Part model, mm, in its own coordinate system. A direction names the side the tool comes from. Round coordinates to 2 decimals unless told otherwise and drop trailing zeros. Order: outer loops, then holes, each group sorted by start corner. A loop starts at its lowest first (then second) coordinate and runs counter-clockwise, first axis right, second up. Notation, with made-up numbers: (-36, 13.5) - (2, 13.5) arc R13 ccw to (2, 17.5) - close; hole circle Ø10 at (21, -1). An arc over 180 degrees is marked (long way). Return JSON: item names as keys, results as strings. Group by question number.
Item 1: Saw through at B-B on z = -0.85. State how many separate pieces and enclosed holes the cut face has, and give its area (3 significant figures).
Item 2: Tool access for faces 5 (the face through (33, 0, -1.25)), 6 (the face through (78.29, 10.97, -0.02)): list every direction of +Z, -Z, +X, -X, +Y, -Y with a clear straight run to the whole face (end or side of a thin tool).
Item 3: Saw through at A-A on x = 100. List the corners of the cut face in (y, z), and give its area (3 significant figures).
Item 4: Probe probe 1 along X at (y, z) = (-7, -0.4); probe 2 along X at (y, z) = (-4, 0.95); probe 3 along Y at (x, z) = (108.5, -0.45). List the from-to ranges inside material, lowest first.
Item 5: Two-plate mould, pull along X, no slides. Class faces 1 (the face through (78.29, -10.97, -0.02)), 2 (the face through (-111.108, -0.319, 0.018)), 3 (the face through (4, 0, 1.25)), 4 (the face through (122.487, 0.771, 0.018)): released by +X, released by -X, zero draft, split by the parting line, or undercut.
Item 6: Drop flat-ended pins along their axis: pin 1 (2.5 mm diameter, centred on x = -96.83, y = 5.5, fed in from +Z); pin 2 (1 mm diameter, centred on x = 46, z = -1, fed in from -Y). Give the stop position or say it passes through.
```python
from build123d import *

# Parameters (mm, degrees)
BOSS_EXTRUDE1_DEPTH      = 1.25000004
FILLET1_R                = 12.7
BOSS_EXTRUDE2_DEPTH      = 1.25000004
SKETCH3_R                = 12
CUT_EXTRUDE1_DEPTH       = 2.25000004
CUT_EXTRUDE1_DEPTH_BACK  = 2.25000004
SKETCH5_R                = 1.500000048
CUT_EXTRUDE2_DEPTH       = 2.25000004
CIRPATTERN1_COUNT        = 6
SKETCH6_R                = 1.500000048
CUT_EXTRUDE3_DEPTH       = 1
CUT_EXTRUDE3_DEPTH_BACK  = 3.50000008
M3_CLEARANCE_HOLE1_D     = 3.4
M3_CLEARANCE_HOLE1_DEPTH = 2.50100008
CIRPATTERN3_COUNT        = 6


with BuildPart() as part:
    # Sketch1 → Boss-Extrude1 (new body, symmetric)
    with BuildSketch(Plane.XY):
        with BuildLine():
            Line((-92.723443504, 8.398772615), (79.761952414, 9.832162885))
            ThreePointArc((79.761952414, 9.832162885), (122.499999983, 0), (79.761952414, -9.832162885))
            Line((79.761952414, -9.832162885), (-92.723443504, -8.398772615))
            ThreePointArc((-92.723443504, -8.398772615), (-111.112500025, 0), (-92.723443504, 8.398772615))
        make_face()
        with BuildLine():
            Line((-88.989202767, 1.5), (77.685740638, 2.885104175))
            ThreePointArc((77.685740638, 2.885104175), (77.500000067, 0), (77.685740638, -2.885104175))
            Line((77.685740638, -2.885104175), (-88.989202767, -1.5))
            Line((-88.989202767, -1.5), (-88.989202767, 1.5))
        make_face(mode=Mode.SUBTRACT)
    extrude(amount=BOSS_EXTRUDE1_DEPTH, both=True)

    # Fillet1
    fillet1_edges = [part.edges().sort_by_distance(p)[0] for p in [
        (-92.723443504, 8.398772615, 0),
        (79.761952414, 9.832162885, 0),
        (79.761952414, -9.832162885, 0),
        (-92.723443504, -8.398772615, 0),
    ]]
    fillet(fillet1_edges, radius=FILLET1_R)

    # Sketch2 → Boss-Extrude2 (add, symmetric)
    with BuildSketch(Plane.XY):
        with BuildLine():
            Line((-88.989202767, 1.5), (-88.989202767, -1.5))
            Line((-88.989202767, -1.5), (77.685740638, -2.885104175))
            ThreePointArc((77.685740638, -2.885104175), (77.500000067, 0), (77.685740638, 2.885104175))
            Line((77.685740638, 2.885104175), (-88.989202767, 1.5))
        make_face()
    extrude(amount=BOSS_EXTRUDE2_DEPTH, both=True)

    # Sketch3 → Cut-Extrude1 (cut, two sides)
    with BuildSketch(Plane.XY) as cut_extrude1_sk:
        with Locations((100.000000025, 0)):
            Circle(SKETCH3_R)
    extrude(amount=CUT_EXTRUDE1_DEPTH, mode=Mode.SUBTRACT)
    extrude(cut_extrude1_sk.sketch, amount=-CUT_EXTRUDE1_DEPTH_BACK, mode=Mode.SUBTRACT)

    # Sketch5 → Cut-Extrude2 (cut, symmetric)
    with BuildSketch(Plane.XY):
        with Locations((116.000000029, 0)):
            Circle(SKETCH5_R)
    cut_extrude2 = extrude(amount=CUT_EXTRUDE2_DEPTH, both=True, mode=Mode.SUBTRACT)

    # CirPattern1: Cut-Extrude2 ×6 about axis
    cirpattern1_axis = Axis((100.000000025, 0, 0), (0, 0, 1))
    for i in range(1, CIRPATTERN1_COUNT):
        add(cut_extrude2.rotate(cirpattern1_axis, i * 360 / CIRPATTERN1_COUNT), mode=Mode.SUBTRACT)

    # Sketch6 → Cut-Extrude3 (cut, two sides)
    with BuildSketch(Plane.XY.offset(1.25000004)) as cut_extrude3_sk:
        with Locations((68.250000025, 0)):
            Circle(SKETCH6_R)
        with Locations((57.137500025, 0)):
            Circle(SKETCH6_R)
        with Locations((46.025000025, 0)):
            Circle(SKETCH6_R)
        with Locations((34.912500025, 0)):
            Circle(SKETCH6_R)
        with Locations((23.800000025, 0)):
            Circle(SKETCH6_R)
        with Locations((12.687500025, 0)):
            Circle(SKETCH6_R)
        with Locations((1.575000025, 0)):
            Circle(SKETCH6_R)
        with Locations((-9.537499975, 0)):
            Circle(SKETCH6_R)
        with Locations((-20.649999975, 0)):
            Circle(SKETCH6_R)
        with Locations((-31.762499975, 0)):
            Circle(SKETCH6_R)
        with Locations((-42.874999975, 0)):
            Circle(SKETCH6_R)
        with Locations((-53.987499975, 0)):
            Circle(SKETCH6_R)
        with Locations((-65.099999975, 0)):
            Circle(SKETCH6_R)
        with Locations((-76.212499975, 0)):
            Circle(SKETCH6_R)
        with Locations((-87.324999975, 0)):
            Circle(SKETCH6_R)
    extrude(amount=CUT_EXTRUDE3_DEPTH, mode=Mode.SUBTRACT)
    extrude(cut_extrude3_sk.sketch, amount=-CUT_EXTRUDE3_DEPTH_BACK, mode=Mode.SUBTRACT)

    # M3 Clearance Hole1
    with Locations(Plane(origin=(0, 0, -1.25000004), x_dir=(-1, 0, 0), z_dir=(0, 0, -1))):
        with Locations((93.650000025, 0)):
            m3_clearance_hole1 = Hole(M3_CLEARANCE_HOLE1_D / 2, depth=M3_CLEARANCE_HOLE1_DEPTH)

    # CirPattern3: M3 Clearance Hole1 ×6 about axis
    cirpattern3_axis = Axis((-100.000000025, 0, 0), (0, 0, 1))
    for i in range(1, CIRPATTERN3_COUNT):
        add(m3_clearance_hole1.rotate(cirpattern3_axis, i * 360 / CIRPATTERN3_COUNT), mode=Mode.SUBTRACT)


solid = part.part
```
Filled in:
{
 "1": {"separate pieces": "1", "enclosed holes": "28", "area": "4,410 mm^2"},
 "2": {"face 5": "-Z, +X, -X, +Y, -Y", "face 6": "+Z, -Z, +Y"},
 "3": {"outline": "(-22.5, -1.25) - (-12, -1.25) - (-12, 1.25) - (-22.5, 1.25) - close; (12, -1.25) - (22.5, -1.25) - (22.5, 1.25) - (12, 1.25) - close", "area": "52.5 mm^2"},
 "4": {"probe 1": "x = -108.63 to -103.97, -102.38 to -97.62, -96.03 to 90.25, 109.75 to 121.38", "probe 2": "x = -110.37 to -103.98, -102.37 to -97.63, -96.02 to 88.69, 111.31 to 122.14", "probe 3": "y = -20.83 to -15.27, -12.44 to -8.47, 8.47 to 12.44, 15.27 to 20.83"},
 "5": {"face 1": "undercut", "face 2": "undercut", "face 3": "zero draft", "face 4": "split by the parting line"},
 "6": {"pin 1": "passes through", "pin 2": "stops at y = -9.56"}
}
